CAD build for the part. Positions are in the model's coordinates, mm. Round coordinates to 2 decimals unless told otherwise and drop trailing zeros. Loops run counter-clockwise (first coordinate to the right, second up) from the corner with the lowest first, then second, coordinate; pieces in that order, holes last. Notation, with made-up numbers: M 25.5,-32.5 L 61.5,-32.5 A6 cw 61.5,-21.5 Z; hole C -23.5,-4.5 d10. An arc over 180 degrees is marked long. Use a Markdown table: item, result. Add a question column.
(1) Band-saw the part on A-A, the plane x = 110. Write the cut outline in (y, z) (1 decimal), and give its area (3 significant figures).
(2) Wall check: L1, parallel to Z at x = 303, y = 0; L2, parallel to Z at x = 165, y = -3.5; L3, parallel to X at y = -8, z = 7. Give the ranges that are in metal, low to high.
(3) Flat gauge pins, fed straight in: P1, Ø1, axis at x = 231.5, y = -6, coming from the -Z side; P2, Ø4, axis at y = 0, z = 0, coming from the +X side; P3, Ø8, axis at x = 175.5, y = -7.5, coming from the -Z side. Where does each tip first touch, or does it go through?
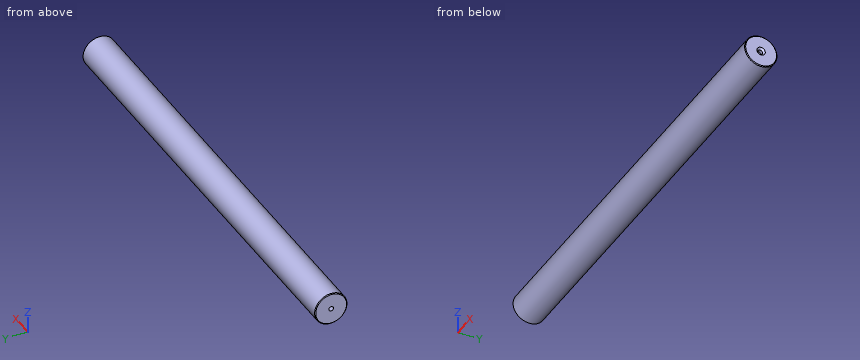
from build123d import *

# Parameters (mm, degrees)
F0_R     = 11.1125
F1_DEPTH = 304.8
F2_R     = 1.5875
F3_DEPTH = 3.175
F4_R     = 1.5875
F5_DEPTH = 5.715
F6_SIZE  = 0.508
F7_SIZE  = 1.27


with BuildPart() as f1:
    # F0 (on Right) → F1 (new body)
    with BuildSketch(Plane.YZ):
        Circle(F0_R)
    extrude(amount=F1_DEPTH)

    # F2 (on face) → F3 (cut)
    with BuildSketch(Plane.YZ.offset(304.8)):
        Circle(F2_R)
    extrude(amount=-F3_DEPTH, mode=Mode.SUBTRACT)

    # F4 (on face) → F5 (cut)
    with BuildSketch(Plane(origin=(0, 0, 0), x_dir=(0, -1, 0), z_dir=(-1, 0, 0))):
        Circle(F4_R)
    extrude(amount=-F5_DEPTH, mode=Mode.SUBTRACT)

    # F6
    f6_edges = [f1.edges().sort_by_distance(p)[0] for p in [
        (0, -11.1125, 0),
        (304.8, -11.1125, 0),
    ]]
    chamfer(f6_edges, length=F6_SIZE)

    # F7
    f7_edges = [f1.edges().sort_by_distance(p)[0] for p in [
        (304.8, -1.5875, 0),
        (5.715, 1.5875, 0),
    ]]
    chamfer(f7_edges, length=F7_SIZE)


solid = f1.part
Return value:
| question | item | result |
|---|---|---|
| 1 | outline | C 0,0 d22.2 |
| 1 | area | 388 mm^2 |
| 2 | L1 | -11.11 to -1.59, 1.59 to 11.11 |
| 2 | L2 | -10.55 to 10.55 |
| 2 | L3 | 0.03 to 304.77 |
| 3 | P1 | z = -9.66 |
| 3 | P2 | x = 303.94 |
| 3 | P3 | z = -10.55 |
